For this review, use the dimensioned drawing (mm, ordinates from the lowest corner) and the shaded views. Round coordinates to 2 decimals unless told otherwise and drop trailing zeros. Order: outer loops, then holes, each group sorted by start corner. A loop starts at its lowest first (then second) coordinate and runs counter-clockwise, first axis right, second up. Notation, with made-up numbers: (-10, -11.5) -> (49, -11.5) arc R33 ccw to (49, 19.5) -> close; hole circle Ø7 at (-37.5, 28). An arc over 180 degrees is marked (long way). Use a Markdown table: item, result. Add a question column.
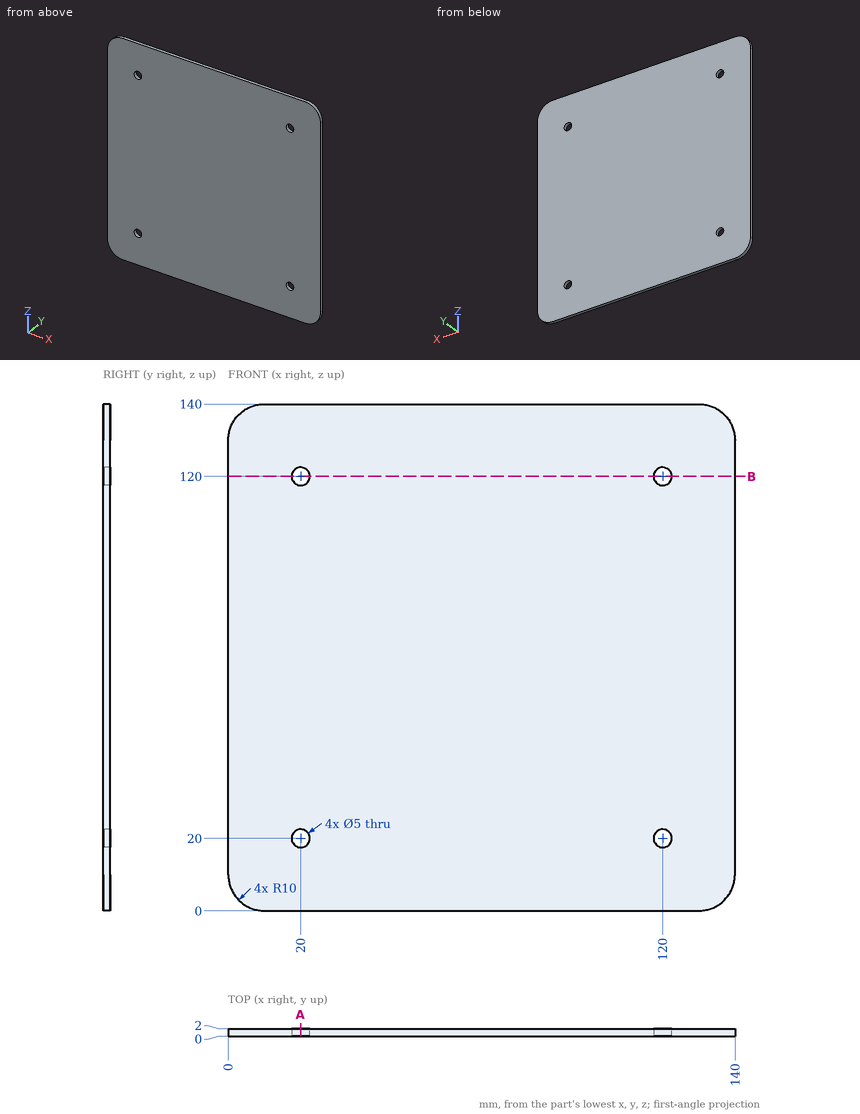
Q1. Add section A-A (x = 20). Write out the cut boundary in (y, z), then the cut area to 3 significant figures.
Q2. Wall thickness on line 1 (Z direction, x = 120, y = 0.5); line 2 (X direction, y = 0.95, z = 21.5): over which ranges is each line inside the solid? List them lowest first. Write a range as [from, to].
Q3. Add section B-B (z = 120). Write out the cut boundary in (x, y), then the cut area to 3 significant figures.
Report:
| question | item | result |
|---|---|---|
| 1 | outline | (0, 0) -> (2, 0) -> (2, 17.5) -> (0, 17.5) -> close; (0, 22.5) -> (2, 22.5) -> (2, 117.5) -> (0, 117.5) -> close; (0, 122.5) -> (2, 122.5) -> (2, 140) -> (0, 140) -> close |
| 1 | area | 260 mm² |
| 2 | line 1 | z = [0, 17.5], [22.5, 117.5], [122.5, 140] |
| 2 | line 2 | x = [0, 18], [22, 118], [122, 140] |
| 3 | outline | (0, 0) -> (17.5, 0) -> (17.5, 2) -> (0, 2) -> close; (22.5, 0) -> (117.5, 0) -> (117.5, 2) -> (22.5, 2) -> close; (122.5, 0) -> (140, 0) -> (140, 2) -> (122.5, 2) -> close |
| 3 | area | 260 mm² |
